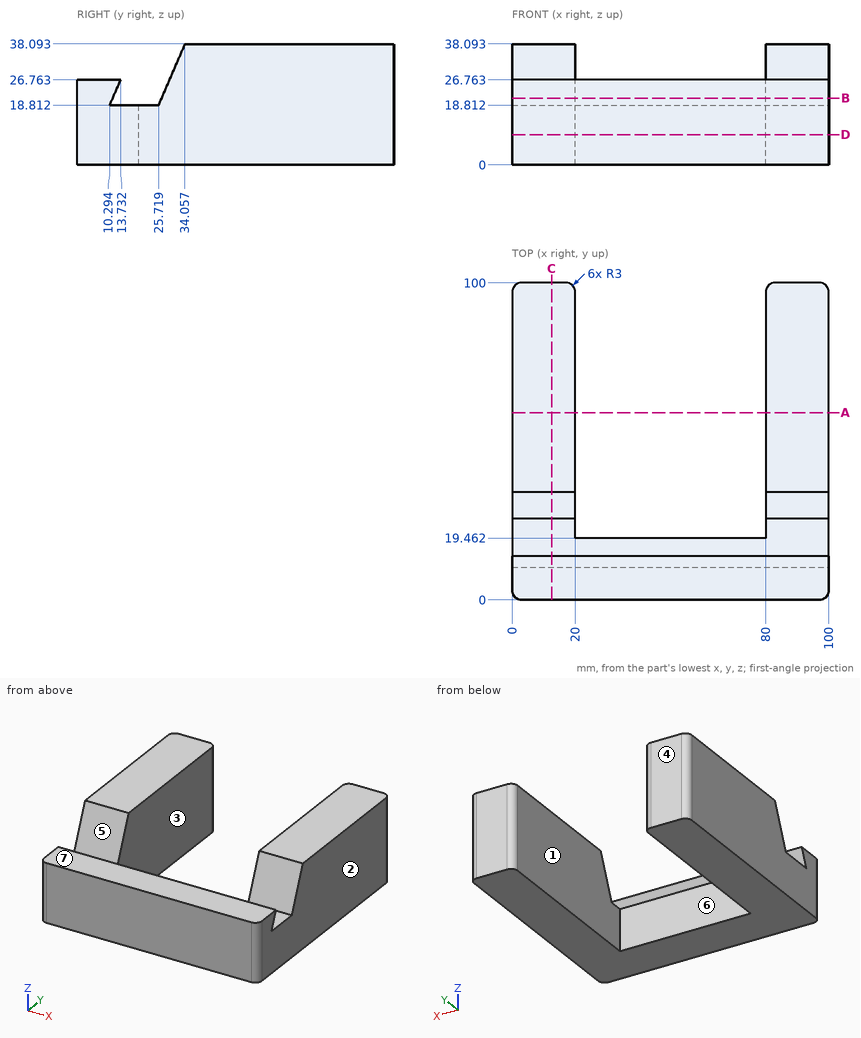
Geometry: see drawing. Coordinates: mm, zero at the bounding-box minimum. A direction names the side the tool comes from. Give positions to 0.01 mm unless a question says otherwise; leave off trailing zeros. Order: outer loops, then holes, each group sorted by start corner. A loop starts at its lowest first (then second) coordinate and runs counter-clockwise, first axis right, second up. Notation, with made-up numbers: (30, -2.75) -> (72, -2.75) arc R37 ccw to (72, 35.25) -> close; hole circle Ø4 at (20, 22.25). An arc over 180 degrees is marked (long way). Write item = value, one per line.
Q1. Cut plane B-B, the plane z = 21. Output: boundary loops of the cut face in (x, y) (1 decimal), and give its area (3 significant figures).
Data:
outline = (0, 3) arc R3 ccw to (3, 0) -> (97, 0) arc R3 ccw to (100, 3) -> (100, 11.2) -> (0, 11.2) -> close; (0, 26.7) -> (20, 26.7) -> (20, 97) arc R3 ccw to (17, 100) -> (3, 100) arc R3 ccw to (0, 97) -> close; (80, 26.7) -> (100, 26.7) -> (100, 97) arc R3 ccw to (97, 100) -> (83, 100) arc R3 ccw to (80, 97) -> close
area = 4,050 mm^2
Q2. Cut plane A-A, the plane y = 59. Output: boundary loops of the cut face in (x, z).
Data:
outline = (0, 0) -> (20, 0) -> (20, 38.09) -> (0, 38.09) -> close; (80, 0) -> (100, 0) -> (100, 38.09) -> (80, 38.09) -> close
Q3. Material intervals for line 1 (X direction, y = 90, z = 25); line 2 (Z direction, x = 18.5, y = 23.5); line 3 (Y direction, x = 66, z = 4), sorted ascending. Write a range as from..to.
Data:
line_1 = 0..20, 80..100
line_2 = 0..18.81
line_3 = 0..19.46
Q4. Cut plane D-D, the plane z = 9.5. Output: boundary loops of the cut face in (x, y), and give its area (3 significant figures).
Data:
outline = (0, 3) arc R3 ccw to (3, 0) -> (97, 0) arc R3 ccw to (100, 3) -> (100, 97) arc R3 ccw to (97, 100) -> (83, 100) arc R3 ccw to (80, 97) -> (80, 19.46) -> (20, 19.46) -> (20, 97) arc R3 ccw to (17, 100) -> (3, 100) arc R3 ccw to (0, 97) -> close
area = 5,160 mm^2
Q5. Cut plane C-C, the plane x = 12.5. Output: boundary loops of the cut face in (y, z) (1 decimal), and give its area (3 significant figures).
Data:
outline = (0, 0) -> (100, 0) -> (100, 38.1) -> (34.1, 38.1) -> (25.7, 18.8) -> (10.3, 18.8) -> (13.7, 26.8) -> (0, 26.8) -> close
area = 3,330 mm^2
Q6. Pin query (flat end, axial travel): pin 1 (4.5 mm diameter, centred on x = 56.5, y = 15, fed in from +Z); pin 2 (15 mm diameter, centred on x = 40, z = 12, fed in from +Y); pin 3 (8 mm diameter, centred on x = 26, z = 30.5, fed in from +Y). Return the tip coordinate at first contact, or that it passes through.
Data:
pin_1 = 26.76
pin_2 = 19.46
pin_3 = 13.73
Q7. Pull-direction query (X, two-part tool) for the marked faces 1, 2, 3 and 4; classes: released by +X, released by -X, zero draft, split by the parting line, or undercut.
Data:
face_1 = undercut
face_2 = released by +X
face_3 = undercut
face_4 = zero draft
Q8. Set-up query: the marked faces 5, 6 and 7. Return all of +Z, -Z, +X, -X, +Y, -Y with unobstructed straight access to the full face (end or side cutting, diameter ignored); none if empty.
Data:
face_5 = +Z, +X, -X
face_6 = +Z, -Z, +Y
face_7 = +Z, +X, -X, -Y
